```python
from build123d import *

# Parameters (mm, degrees)
SKETCH1_W           = 200
SKETCH1_H           = 140
BOSS_EXTRUDE1_DEPTH = 3
FILLET1_R           = 15
BOSS_EXTRUDE2_DEPTH = 6
SKETCH4_R           = 4
CUT_EXTRUDE1_DEPTH  = 2
SKETCH5_R           = 1.85
CUT_EXTRUDE2_DEPTH  = 6
SKETCH6_R           = 4
CUT_EXTRUDE3_DEPTH  = 2
SKETCH7_R           = 1.85
CUT_EXTRUDE4_DEPTH  = 2


with BuildPart() as part:
    # Sketch1 → Boss-Extrude1 (new body)
    with BuildSketch(Plane(origin=(0, 0, 0), x_dir=(1, 0, 0), z_dir=(0, 1, 0))):
        Rectangle(SKETCH1_W, SKETCH1_H)
    extrude(amount=BOSS_EXTRUDE1_DEPTH)

    # Fillet1
    fillet1_edges = [part.edges().sort_by_distance(p)[0] for p in [
        (100, 1.5, 70),
        (-100, 1.5, 70),
        (-100, 1.5, -70),
        (100, 1.5, -70),
    ]]
    fillet(fillet1_edges, radius=FILLET1_R)

    # Sketch3 → Boss-Extrude2 (add)
    with BuildSketch(Plane(origin=(0, 3, 0), x_dir=(1, 0, 0), z_dir=(0, 1, 0))):
        with BuildLine():
            Line((96, -55), (96, 55))
            ThreePointArc((96, 55), (92.778174593, 62.778174593), (85, 66))
            Line((85, 66), (-85, 66))
            ThreePointArc((-85, 66), (-92.778174593, 62.778174593), (-96, 55))
            Line((-96, 55), (-96, -55))
            ThreePointArc((-96, -55), (-92.778174593, -62.778174593), (-85, -66))
            Line((-85, -66), (85, -66))
            ThreePointArc((85, -66), (92.778174593, -62.778174593), (96, -55))
        make_face()
        with BuildLine():
            Line((85, 63), (-85, 63))
            ThreePointArc((-85, 63), (-90.656854249, 60.656854249), (-93, 55))
            Line((-93, 55), (-93, -55))
            ThreePointArc((-93, -55), (-90.656854249, -60.656854249), (-85, -63))
            Line((-85, -63), (85, -63))
            ThreePointArc((85, -63), (90.656854249, -60.656854249), (93, -55))
            Line((93, -55), (93, 55))
            ThreePointArc((93, 55), (90.656854249, 60.656854249), (85, 63))
        make_face(mode=Mode.SUBTRACT)
    extrude(amount=BOSS_EXTRUDE2_DEPTH)

    # Sketch4 → Cut-Extrude1 (cut)
    with BuildSketch(Plane(origin=(0, 0, 0), x_dir=(-1, 0, 0), z_dir=(0, -1, 0))):
        with Locations((82.73, -55.7)):
            Circle(SKETCH4_R)
    cut_extrude1 = extrude(amount=-CUT_EXTRUDE1_DEPTH, mode=Mode.SUBTRACT)

    # Mirror1: Cut-Extrude1 across plane
    add(cut_extrude1.mirror(Plane.XY), mode=Mode.SUBTRACT)

    # Sketch5 → Cut-Extrude2 (cut)
    with BuildSketch(Plane.XZ.offset(-2)):
        with Locations((-82.73, 55.7)):
            Circle(SKETCH5_R)
    cut_extrude2 = extrude(amount=-CUT_EXTRUDE2_DEPTH, mode=Mode.SUBTRACT)

    # Mirror2: Cut-Extrude2 across plane
    add(cut_extrude2.mirror(Plane.XY), mode=Mode.SUBTRACT)

    # Sketch6 → Cut-Extrude3 (cut)
    with BuildSketch(Plane(origin=(0, 0, 0), x_dir=(-1, 0, 0), z_dir=(0, -1, 0))):
        with Locations((-82, -55.25)):
            Circle(SKETCH6_R)
    cut_extrude3 = extrude(amount=-CUT_EXTRUDE3_DEPTH, mode=Mode.SUBTRACT)

    # Mirror3: Cut-Extrude3 across plane
    add(cut_extrude3.mirror(Plane.XY), mode=Mode.SUBTRACT)

    # Sketch7 → Cut-Extrude4 (cut)
    with BuildSketch(Plane(origin=(0, 2, 0), x_dir=(-1, 0, 0), z_dir=(0, -1, 0))):
        with Locations((-82, -55.25)):
            Circle(SKETCH7_R)
    cut_extrude4 = extrude(amount=-CUT_EXTRUDE4_DEPTH, mode=Mode.SUBTRACT)

    # Mirror4: Cut-Extrude4 across plane
    add(cut_extrude4.mirror(Plane.XY), mode=Mode.SUBTRACT)


solid = part.part
```
CAD build for the part. Positions are in the model's coordinates, mm. A direction names the side the tool comes from. Round coordinates to 2 decimals unless told otherwise and drop trailing zeros. Loops run counter-clockwise (first coordinate to the right, second up) from the corner with the lowest first, then second, coordinate; pieces in that order, holes last. Notation, with made-up numbers: (58.5, 60) - (96.5, 60) arc R19 ccw to (96.5, 71) - close; hole circle Ø5 at (21, 5). An arc over 180 degrees is marked (long way). Return JSON: item names as keys, results as strings. Group by question number.
Q1. Tool access for faces 5 (the face through (-90.594, 5.958, -60.719)), 6 (the face through (-95.72, 1.52, 65.49)), 7 (the face through (-81, 2, 57)), 8 (the face through (-80.965, 2.493, 56.256)), 9 (the face through (96, 6, 1)): list every direction of +Z, -Z, +X, -X, +Y, -Y with a clear straight run to the whole face (end or side of a thin tool).
Q2. Drill centre lines: line 1 along Z through (x, y) = (-82.73, 0.75); line 2 along Z through (x, y) = (82, 1.5); line 3 along X through (y, z) = (1.1, 55.7). Where is each one in solid material? Low to high. Write a range as [from, to].
Q3. Band-saw the part on B-B on z = -28. Give the cut face in (x, y).
Q4. Two-plate mould, pull along Z, no slides. Class faces 1 (the face through (-80.965, 2.493, -56.256)), 2 (the face through (-86.425, 0.986, 57.232)), 3 (the face through (-1, 6, 66)), 4 (the face through (-95.72, 1.52, -65.49)): +Z half, -Z half, draft (parallel to the pull), parting line (faces both ways), or undercut.
Q5. Flat gauge pins, fed straight in: pin 1 Ø3 at (x, y) = (53, 6.5) entering from +Z; pin 2 Ø3.5 at (x, z) = (82, -55.25) entering from +Y; pin 3 Ø4 at (x, z) = (-82, -55) entering from -Y; pin 4 Ø10 at (x, z) = (-53.5, -2.5) entering from +Y. Where does each tip first touch, or does it go through?
Q6. Band-saw the part on A-A on x = 69.5. Give the cut face in (y, z), plus the area to 3 significant figures.
Solutions:
{
 "1": {"face 5": "+Y", "face 6": "+Z, -X, +Y, -Y", "face 7": "-Y", "face 8": "+Y, -Y", "face 9": "+Z, -Z, +X, +Y"},
 "2": {"line 1": "z = [-70, -59.7], [-51.7, 51.7], [59.7, 70]", "line 2": "z = [-70, -59.25], [-51.25, 51.25], [59.25, 70]", "line 3": "x = [-99.98, -86.73], [-78.73, 78.03], [85.97, 99.98]"},
 "3": {"outline": "(-100, 0) - (100, 0) - (100, 3) - (96, 3) - (96, 9) - (93, 9) - (93, 3) - (-93, 3) - (-93, 9) - (-96, 9) - (-96, 3) - (-100, 3) - close"},
 "4": {"face 1": "undercut", "face 2": "undercut", "face 3": "+Z half", "face 4": "-Z half"},
 "5": {"pin 1": "stops at z = 66", "pin 2": "passes through", "pin 3": "stops at y = 2", "pin 4": "stops at y = 3"},
 "6": {"outline": "(0, -70) - (3, -70) - (3, -66) - (9, -66) - (9, -63) - (3, -63) - (3, 63) - (9, 63) - (9, 66) - (3, 66) - (3, 70) - (0, 70) - close", "area": "456 mm^2"}
}
